Study the drawing (mm; zero at the part's minimum x, y, z) and answer. A direction names the side the tool comes from. Round coordinates to 2 decimals unless told otherwise and drop trailing zeros. Loops run counter-clockwise (first coordinate to the right, second up) from the corner with the lowest first, then second, coordinate; pieces in that order, holes last. Notation, with made-up numbers: M 83.5,5 L 135.5,5 A25 ccw 135.5,35 Z; hole C 66,-24 d7. An arc over 180 degrees is marked long. Write each question's results on one line, items separated by ' | '.
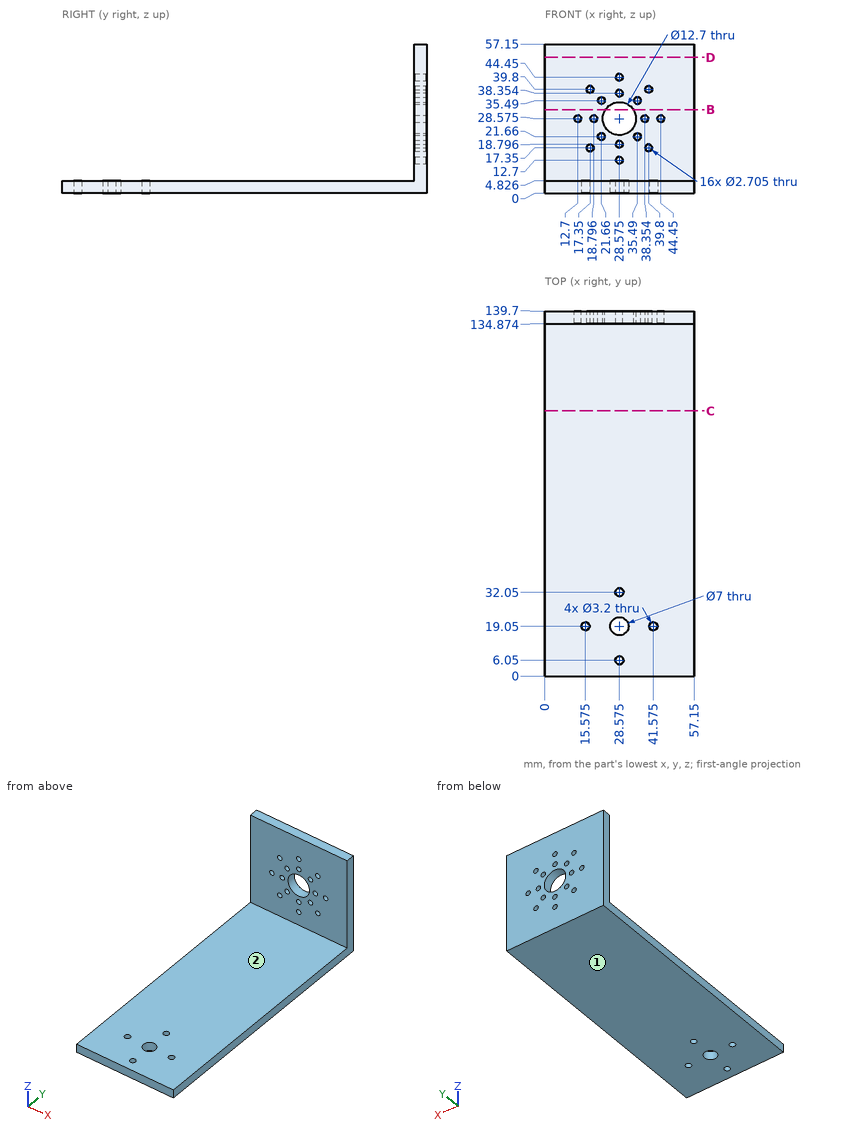
Item 1: The part is cut by section B-B (z = 32). Determine the outline of the cut face in (x, y), plus the area to 3 significant figures.
Outcome:
outline: M 0,134.87 L 23.23,134.87 L 23.23,139.7 L 0,139.7 Z; M 33.92,134.87 L 57.15,134.87 L 57.15,139.7 L 33.92,139.7 Z | area: 224 mm2
Item 2: The part is cut by section D-D (z = 52). Determine the outline of the cut face in (x, y).
Outcome:
outline: M 0,134.87 L 57.15,134.87 L 57.15,139.7 L 0,139.7 Z
Item 3: For the marked faces 1 and 2, determine the directions among +Z, -Z, +X, -X, +Y, -Y from which every point of the face is accessible in a straight line to the end or side of a thin tool.
Outcome:
face 1: -Z, +X, -X, +Y, -Y | face 2: +Z, +X, -X, -Y
Item 4: Flat-ended cylindrical pins translate along their axes: pin 1 (20.5 mm diameter, centred on x = 28.575, z = 28.575, fed in from +Y); pin 2 (4.5 mm diameter, centred on x = 39.8, z = 17.35, fed in from -Y). Find the tip coordinate at first contact, or state that the pin passes through.
Outcome:
pin 1: stops at y = 139.7 | pin 2: stops at y = 134.87
Item 5: The part is cut by section C-C (y = 101.5). Determine the outline of the cut face in (x, z), plus the area to 3 significant figures.
Outcome:
outline: M 0,0 L 57.15,0 L 57.15,4.83 L 0,4.83 Z | area: 276 mm2
Item 6: Straight lines are drawn through the part: line 1 (Z direction, x = 12.7, y = 136.85); line 2 (Z direction, x = 38.5, y = 17); line 3 (Y direction, x = 17, z = 42). For each, find the intervals that lie inside material, in ascending order.
Outcome:
line 1: z = 0 to 27.22, 29.93 to 57.15 | line 2: z = 0 to 4.83 | line 3: y = 134.87 to 139.7
